```python
from build123d import *

# Parameters (mm, degrees)
F1_DEPTH = 3
F2_R     = 13.5
F2_R_2   = 10
F3_DEPTH = 2
F4_DEPTH = 1
F5_R     = 10.2
F5_R_2   = 10
F6_DEPTH = 25


with BuildPart() as f1:
    # F0 (on Top) → F1 (new body)
    with BuildSketch(Plane.XY):
        with BuildLine():
            ThreePointArc((35, 0), (10.4809717311, 33.3938502059), (-28.7228132327, 20))
            Line((-28.7228132327, 20), (20, 20))
            Line((20, 20), (20, -20))
            Line((20, -20), (-28.7228132327, -20))
            ThreePointArc((-28.7228132327, -20), (10.4809717311, -33.3938502059), (35, 0))
        make_face()
        with BuildLine():
            ThreePointArc((-28.7228132327, 20), (-33.3938502059, 10.4809717311), (-35, 0))
            ThreePointArc((-35, 0), (-33.3938502059, -10.4809717311), (-28.7228132327, -20))
            Line((-28.7228132327, -20), (20, -20))
            Line((20, -20), (20, 20))
            Line((20, 20), (-28.7228132327, 20))
        make_face()
        with BuildLine():
            ThreePointArc((-10, 0), (0, 10), (10, 0))
            ThreePointArc((10, 0), (0, -10), (-10, 0))
        make_face(mode=Mode.SUBTRACT)
    extrude(amount=F1_DEPTH)

    # F2 (on face) → F3 (join)
    with BuildSketch(Plane(origin=(0, 0, 0), x_dir=(1, 0, 0), z_dir=(0, 0, -1))):
        Circle(F2_R)
        Circle(F2_R_2, mode=Mode.SUBTRACT)
    extrude(amount=F3_DEPTH)

    # F4 (cut): a face of the model
    f4_faces = [f1.faces().sort_by_distance(p)[0] for p in [
        (-34.0100505063, 0, 3),
    ]]
    extrude(f4_faces, amount=-F4_DEPTH, mode=Mode.SUBTRACT)

    # F5 (on face) → F6 (cut)
    with BuildSketch(Plane.XY.offset(2)):
        Circle(F5_R)
        Circle(F5_R_2, mode=Mode.SUBTRACT)
    extrude(amount=-F6_DEPTH, mode=Mode.SUBTRACT)


solid = f1.part
```
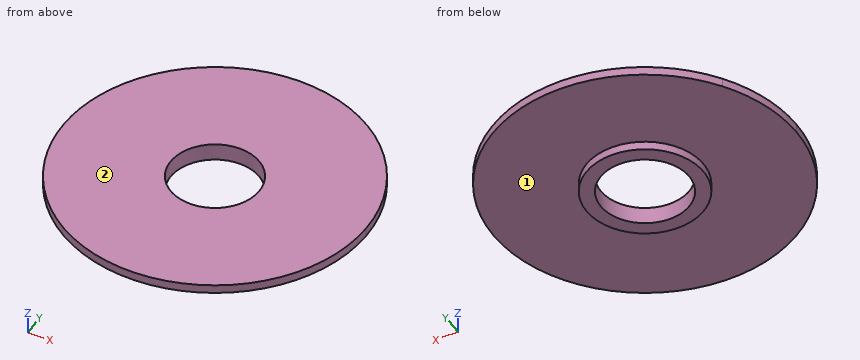
CAD build for the part. Positions are in the model's coordinates, mm. Face numbers are marked on the shaded views. A direction names the side the tool comes from. Coordinates: 2 decimals unless noted, no trailing zeros. Order: outer loops, then holes, each group sorted by start corner. A loop starts at its lowest first (then second) coordinate and runs counter-clockwise, first axis right, second up.
(1) Saw through at B-B, the plane y = 11.5. Write the cut outline in (x, z).
Solution:
outline: (-33.06, 0) - (-7.07, 0) - (-7.07, -2) - (7.07, -2) - (7.07, 0) - (33.06, 0) - (33.06, 2) - (-33.06, 2) - close
(2) Saw through at A-A, the plane x = 0. Write the cut outline in (y, z), and give its area (3 significant figures).
Solution:
outline: (-35, 0) - (-13.5, 0) - (-13.5, -2) - (-10.2, -2) - (-10.2, 2) - (-35, 2) - close; (10.2, -2) - (13.5, -2) - (13.5, 0) - (35, 0) - (35, 2) - (10.2, 2) - close
area: 112 mm2
(3) Drill centre lines: L1, parallel to Y at x = 0, z = -1.1; L2, parallel to Y at x = 0, z = 0.7; L3, parallel to Z at x = -31, y = 0. Where is each one in solid material? Low to high.
Solution:
L1: y = -13.5 to -10.2, 10.2 to 13.5
L2: y = -35 to -10.2, 10.2 to 35
L3: z = 0 to 2
(4) Saw through at C-C, the plane z = -1.4. Write the cut outline in (x, y).
Solution:
outline: circle Ø27 at (0, 0); hole circle Ø20.4 at (0, 0)
(5) Pin check, flat tips, straight feed: pin 1 Ø3 at (x, y) = (-19.5, -27.5) entering from -Z; pin 2 Ø1.5 at (y, z) = (-23, -0.5) entering from +X; pin 3 Ø23.5 at (x, y) = (0, 0) entering from +Z; pin 4 Ø2 at (x, z) = (27.5, -1.5) entering from -Y. Stop position of each tip, or through.
Solution:
pin 1: stops at z = 0
pin 2: stops at x = 26.86
pin 3: stops at z = 2
pin 4: passes through
(6) Saw through at D-D, the plane x = -11. Write the cut outline in (y, z).
Solution:
outline: (-33.23, 0) - (-7.83, 0) - (-7.83, -2) - (7.83, -2) - (7.83, 0) - (33.23, 0) - (33.23, 2) - (-33.23, 2) - close
(7) Which spindle directions (+Z, -Z, +X, -X, +Y, -Y) get a long thin tool onto all of the face, cutting with end or side? Do the marked faces 1 and 2. Say none if no direction does.
Solution:
face 1: -Z
face 2: +Z, +X, -X, +Y, -Y
